Geometry check sheet. Reference: the model listing, model coordinates, mm. Face numbers are marked on the shaded views. A direction names the side the tool comes from. Round coordinates to 2 decimals unless told otherwise and drop trailing zeros. Loops run counter-clockwise (first coordinate to the right, second up) from the corner with the lowest first, then second, coordinate; pieces in that order, holes last. Notation, with made-up numbers: M 63.5,18.25 L 118.5,18.25 A23 cw 118.5,51.25 Z; hole C 4,12 d3. An arc over 180 degrees is marked long. Write item = value, one per line.
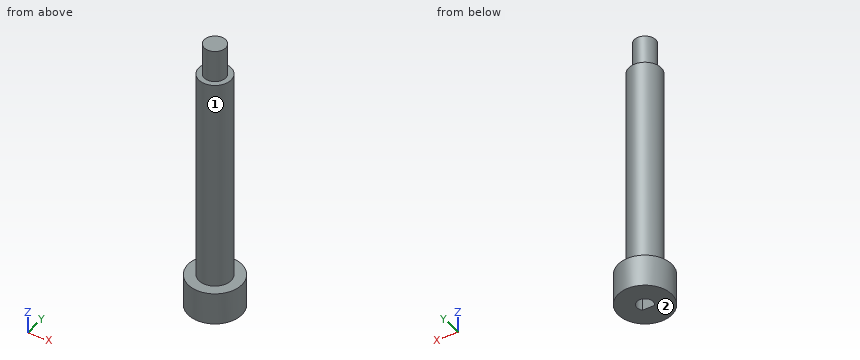
from build123d import *

# Parameters (mm, degrees)
CROQUIS1_R              = 5
SALIENTE_EXTRUIR1_DEPTH = 6
CORTAR_EXTRUIR1_DEPTH   = 5
CROQUIS3_R              = 3
SALIENTE_EXTRUIR2_DEPTH = 40
CROQUIS4_R              = 2
SALIENTE_EXTRUIR3_DEPTH = 6


with BuildPart() as part:
    # Croquis1 → Saliente-Extruir1 (new body)
    with BuildSketch(Plane.XY):
        Circle(CROQUIS1_R)
    extrude(amount=SALIENTE_EXTRUIR1_DEPTH)

    # Croquis2 → Cortar-Extruir1 (cut)
    with BuildSketch(Plane(origin=(0, 0, 0), x_dir=(-1, 0, 0), z_dir=(0, 0, -1))):
        with BuildLine():
            Line((-1.118033989, -1), (0, -1))
            Line((0, -1), (0.606924942, -1))
            Line((0.606924942, -1), (1.118033989, -1))
            ThreePointArc((1.118033989, -1), (0, 1.5), (-1.118033989, -1))
        make_face()
    extrude(amount=-CORTAR_EXTRUIR1_DEPTH, mode=Mode.SUBTRACT)

    # Croquis3 → Saliente-Extruir2 (add)
    with BuildSketch(Plane.XY.offset(6)):
        Circle(CROQUIS3_R)
    extrude(amount=SALIENTE_EXTRUIR2_DEPTH)

    # Croquis4 → Saliente-Extruir3 (add)
    with BuildSketch(Plane.XY.offset(46)):
        Circle(CROQUIS4_R)
    extrude(amount=SALIENTE_EXTRUIR3_DEPTH)


solid = part.part
(1) Tool access check on the marked faces 1 and 2. Record the directions out of +Z, -Z, +X, -X, +Y, -Y that give a thin tool (end or side, any length) a straight path to the whole face; none if there is none.
Result set:
face_1 = +Z
face_2 = -Z, +X, -X, +Y, -Y
(2) Sectioned sample at B-B on x = 0. Record the cut outline in (y, z).
Result set:
outline = M -5,0 L -1,0 L -1,5 L 1.5,5 L 1.5,0 L 5,0 L 5,6 L 3,6 L 3,46 L 2,46 L 2,52 L -2,52 L -2,46 L -3,46 L -3,6 L -5,6 Z
(3) Sectioned sample at C-C on z = 48. Record the cut outline in (x, y), then the cut area to 3 significant figures.
Result set:
outline = C 0,0 d4
area = 12.6 mm2
(4) Sectioned sample at A-A on y = 0. Record the cut outline in (x, z), then the cut area to 3 significant figures.
Result set:
outline = M -5,0 L -1.5,0 L -1.5,5 L 1.5,5 L 1.5,0 L 5,0 L 5,6 L 3,6 L 3,46 L 2,46 L 2,52 L -2,52 L -2,46 L -3,46 L -3,6 L -5,6 Z
area = 309 mm2
(5) Material ranges on line 1 along Y through (x, z) = (0, 2.3); line 2 along Z through (x, y) = (-0.5, -0.75); line 3 along Z through (x, y) = (0.25, 4), recorded low to high. Write a range as from..to.
Result set:
line_1 = -5..-1, 1.5..5
line_2 = 5..52
line_3 = 0..6
(6) Sectioned sample at D-D on z = 35. Record the cut outline in (x, y), then the cut area to 3 significant figures.
Result set:
outline = C 0,0 d6
area = 28.3 mm2
(7) Depth check by flat-ended pin: pin 1 Ø1.5 at (x, y) = (-4, -3) entering from +Z; pin 2 Ø5 at (y, z) = (-1, 21) entering from +X. Enter the tip coordinate at first touch or a pass-through.
Result set:
pin_1 = 6
pin_2 = 3
